Here's how the part is built. I have some questions about the finished solid (model axes, mm). Face numbers are marked on the shaded views. A direction names the side the tool comes from. Round coordinates to 2 decimals unless told otherwise and drop trailing zeros. Write each loop counter-clockwise with the first axis right and the second up, starting at its lowest first coordinate (ties: lowest second). Pieces come first, ordered by that corner, then holes. Notation, with made-up numbers: (74, 80) -> (93, 80) arc R35 ccw to (93, 115) -> close; hole circle Ø11 at (23.5, 75.25). An arc over 180 degrees is marked (long way). Answer as CSV lines item,"result".
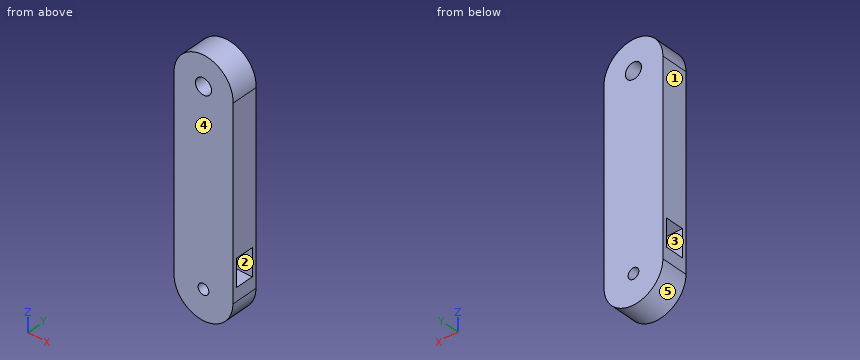
```python
from build123d import *

# Parameters (mm, degrees)
EXTRUDE_START       = -3
EXTRUDE_1_DEPTH     = 3
SKETCH_4_R          = 1
CUT_EXTRUDE_1_DEPTH = 5
EXTRUDE_3_DEPTH     = 2
CUT_EXTRUDE_START   = 10
SKETCH_4_2_R        = 1
CUT_EXTRUDE_2_DEPTH = 10
SKETCH_6_W          = 5.1
SKETCH_6_H          = 3.4
CUT_EXTRUDE_3_DEPTH = 43.585635121


with BuildPart() as part:
    # 草图1 → 旋转1 (revolve)
    with BuildSketch(Plane.XY, mode=Mode.PRIVATE) as revolve_1_sk:
        Polygon((-2.4, 0), (-5.5, 0), (-5.5, 5), (-4.25, 5), (-1.5, 5), (-1.5, 3.8), (-1.5, 2.66), (-1.5, 0), align=None)
    revolve(revolve_1_sk.sketch.rotate(Axis((0, 0, 0), (0, 1, 0)), 270), axis=Axis((0, 0, 0), (0, 1, 0)))

    # 草图2 → 凸台-拉伸1 (add)
    with BuildSketch(Plane(origin=(0, 2, 0), x_dir=(-1, 0, 0), z_dir=(0, -1, 0)).offset(EXTRUDE_START)):
        with BuildLine():
            Line((-5.489247302, 0.34375), (-5.489247302, 35.34375))
            ThreePointArc((-5.489247302, 35.34375), (0.005376349, 40.838373651), (5.5, 35.34375))
            Line((5.5, 35.34375), (5.5, 0))
            ThreePointArc((5.5, 0), (0.171959067, 5.497311168), (-5.489247302, 0.34375))
        make_face()
    extrude(amount=EXTRUDE_1_DEPTH)

    # 草图4 → 切除-拉伸1 (cut, symmetric)
    with BuildSketch(Plane.XZ.offset(-2)):
        with Locations(Location((-0.005376349, -35.34375, 0), (0, 0, 270))):
            Circle(SKETCH_4_R)
    extrude(amount=CUT_EXTRUDE_1_DEPTH, both=True, mode=Mode.SUBTRACT)

    # 草图2<2> → 凸台-拉伸3 (add)
    with BuildSketch(Plane(origin=(0, 2, 0), x_dir=(-1, 0, 0), z_dir=(0, -1, 0))):
        with BuildLine():
            Line((-5.489247302, 0.34375), (-5.489247302, 35.34375))
            ThreePointArc((-5.489247302, 35.34375), (0.005376349, 40.838373651), (5.5, 35.34375))
            Line((5.5, 35.34375), (5.5, 0))
            ThreePointArc((5.5, 0), (0.171959067, 5.497311168), (-5.489247302, 0.34375))
        make_face()
    extrude(amount=EXTRUDE_3_DEPTH)

    # 草图4<2> → 切除-拉伸2 (cut)
    with BuildSketch(Plane.XZ.offset(-2).offset(CUT_EXTRUDE_START)):
        with Locations(Location((-0.005376349, -35.34375, 0), (0, 0, 270))):
            Circle(SKETCH_4_2_R)
    extrude(amount=-CUT_EXTRUDE_2_DEPTH, mode=Mode.SUBTRACT)

    # 草图6 → 切除-拉伸3 (cut, through all)
    with BuildSketch(Plane(origin=(5.489247302, 0, 0), x_dir=(0, 0, -1), z_dir=(1, 0, 0))):
        with Locations((30.34375, 2.5)):
            Rectangle(SKETCH_6_W, SKETCH_6_H)
    extrude(amount=-CUT_EXTRUDE_3_DEPTH, mode=Mode.SUBTRACT)


solid = part.part
```
1. Suppose I cut it at B-B on y = 1.3. Please give me the cut outline in (x, z), and give its area (3 significant figures).
Numbers:
outline,"(-5.5, -35.34) arc R5.49 ccw to (5.49, -35.34) -> (5.49, -32.89) -> (-5.5, -32.89) -> close; (-5.5, -27.79) -> (5.49, -27.79) -> (5.49, -0.34) arc R5.5 ccw (long way) to (-5.5, 0) -> close; hole circle Ø3 at (0, 0); hole circle Ø2 at (-0.01, -35.34)"
area,"417 mm^2"
2. If I drill on line 1 (Y direction, x = 1.75, z = -31.5); line 2 (X direction, y = 2.8, z = 0); line 3 (X direction, y = 4.15, z = -7.5), over which ranges is the centre line in solid material (lowest first)?
Numbers:
line 1,"y = 0 to 0.8, 4.2 to 5"
line 2,"x = -5.5 to -1.5, 1.5 to 5.5"
line 3,"x = -5.5 to 5.49"
3. Suppose I cut it at A-A on z = -29. Please give me the cut outline in (x, y), and give its area (3 significant figures).
Numbers:
outline,"(-5.5, 0) -> (5.49, 0) -> (5.49, 0.8) -> (-5.5, 0.8) -> close; (-5.5, 4.2) -> (5.49, 4.2) -> (5.49, 5) -> (-5.5, 5) -> close"
area,"17.6 mm^2"
4. For pin 1 Ø2.5 at (x, z) = (0, 0) entering from -Y; pin 2 Ø2.5 at (y, z) = (2.5, -23) entering from +X; pin 3 Ø1 at (x, y) = (1, 4.5) entering from +Z; pin 4 Ø2 at (x, y) = (-4, 1) entering from -Z, each with a flat end and sliding along its axis, tell me the tip position at first contact or that it passes through.
Numbers:
pin 1,"passes through"
pin 2,"stops at x = 5.49"
pin 3,"stops at z = 5.48"
pin 4,"stops at z = -39.95"
5. Suppose I cut it at D-D on x = 2. Please give me the cut outline in (y, z), and give its area (3 significant figures).
Numbers:
outline,"(0, -40.46) -> (5, -40.46) -> (5, 5.12) -> (0, 5.12) -> close; hole (0.8, -32.89) -> (4.2, -32.89) -> (4.2, -27.79) -> (0.8, -27.79) -> close"
area,"211 mm^2"
6. Suppose I cut it at C-C on x = 4.75. Please give me the cut outline in (y, z).
Numbers:
outline,"(0, -38.1) -> (5, -38.1) -> (5, 2.77) -> (0, 2.77) -> close; hole (0.8, -32.89) -> (4.2, -32.89) -> (4.2, -27.79) -> (0.8, -27.79) -> close"
7. If we mould it in two halves opening along Z, with no side actions, what happens to the marked faces 3, 4 and 5? For each: released by +Z, released by -Z, zero draft, split by the parting line, or undercut.
Numbers:
face 3,"undercut"
face 4,"zero draft"
face 5,"released by -Z"
8. On a 3-axis mill with a long thin cutter (end or side, diameter ignored), from which of +Z, -Z, +X, -X, +Y, -Y can I reach the whole of each face in a straight line? I mean the marked faces 1 and 2. Say none if no direction works.
Numbers:
face 1,"+Z, -Z, -X, +Y, -Y"
face 2,"+X, -X"
